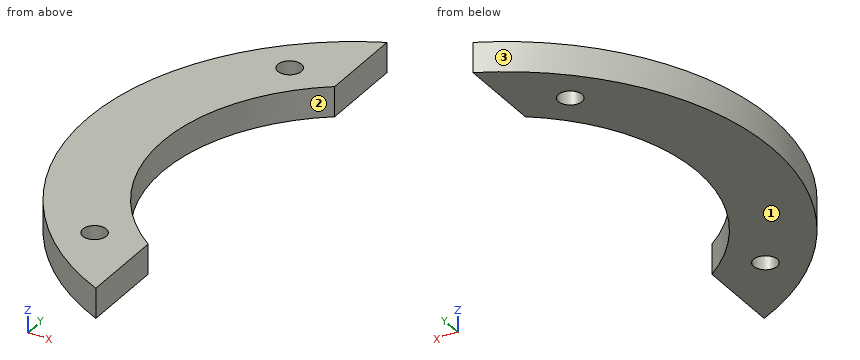
```python
from build123d import *

# Parameters (mm, degrees)
SKETCH_1_R          = 35.5
SKETCH_1_R_2        = 25.5
EXTRUDE_1_DEPTH     = 4
SKETCH_2_R          = 1.575
CUT_EXTRUDE_1_DEPTH = 51.363677388
SKETCH_3_W          = 60
SKETCH_3_H          = 80
CUT_EXTRUDE_2_DEPTH = 51.363677388


with BuildPart() as part:
    # 草图1 → 凸台-拉伸1 (new body)
    with BuildSketch(Plane.XY):
        Circle(SKETCH_1_R)
        Circle(SKETCH_1_R_2, mode=Mode.SUBTRACT)
    extrude(amount=EXTRUDE_1_DEPTH)

    # 草图2 → 切除-拉伸1 (cut, through all)
    with BuildSketch(Plane.XY.offset(4)):
        with Locations((-21.566756826, 21.566756826)):
            Circle(SKETCH_2_R)
        with Locations((21.566756826, 21.566756826)):
            Circle(SKETCH_2_R)
        with Locations((21.566756826, -21.566756826)):
            Circle(SKETCH_2_R)
        with Locations((-21.566756826, -21.566756826)):
            Circle(SKETCH_2_R)
    extrude(amount=-CUT_EXTRUDE_1_DEPTH, mode=Mode.SUBTRACT)

    # 草图3 → 切除-拉伸2 (cut, through all)
    with BuildSketch(Plane.XY.offset(4)):
        with Locations((15, 0)):
            Rectangle(SKETCH_3_W, SKETCH_3_H)
    extrude(amount=-CUT_EXTRUDE_2_DEPTH, mode=Mode.SUBTRACT)


solid = part.part
```
Source: CAD feature listing. Evaluate the final solid. Frame: model axes, mm. Face numbers are marked on the shaded views. Give positions to 0.01 mm unless a question says otherwise; leave off trailing zeros. Write each loop counter-clockwise with the first axis right and the second up, starting at its lowest first coordinate (ties: lowest second). Pieces come first, ordered by that corner, then holes. Notation, with made-up numbers: (67.25, -33) - (74.25, -33) arc R25 ccw to (74.25, 3) - close; hole circle Ø6 at (-9, -34.75). An arc over 180 degrees is marked (long way). One line per item, written item: value. Start each with the question number.
Q1. Section query D-D, the plane x = -28.25. Return the cut outline in (y, z), then the cut area to 3 significant figures.
Q2. Section query B-B, the plane y = 22.5. Return the cut outline in (x, z), then the cut area to 3 significant figures.
Q3. Section query A-A, the plane x = -17. Return the cut outline in (y, z).
Q4. Section query C-C, the plane z = 2.1. Return the cut outline in (x, y) (3 decimals).
Q5. Material intervals for probe 1 along Y at (x, z) = (-17.5, 2.45); probe 2 along X at (y, z) = (22, 2); probe 3 along Y at (x, z) = (-17.25, 3.2), sorted ascending. Write a range as from..to.
Q6. Draft query along Y for the marked faces 1, 2 and 3. Return one class per face: +Y half, -Y half, draft (parallel to the pull), parting line (faces both ways), or undercut.
Q7. First-contact query: pin 1 Ø1 at (x, z) = (-29.5, 2) entering from +Y; pin 2 Ø3 at (x, y) = (-21.57, 21.57) entering from -Z; pin 3 Ø1.5 at (y, z) = (-15.5, 1) entering from +X. Flat tips, straight axial feed; report the tip coordinate or a pass-through.
Answer:
1. outline: (-21.5, 0) - (21.5, 0) - (21.5, 4) - (-21.5, 4) - close
1. area: 172 mm2
2. outline: (-27.46, 0) - (-22.84, 0) - (-22.84, 4) - (-27.46, 4) - close; (-20.3, 0) - (-15, 0) - (-15, 4) - (-20.3, 4) - close
2. area: 39.7 mm2
3. outline: (-31.16, 0) - (-19.01, 0) - (-19.01, 4) - (-31.16, 4) - close; (19.01, 0) - (31.16, 0) - (31.16, 4) - (19.01, 4) - close
4. outline: (-15, -32.175) - (-15, -20.622) arc R25.5 cw to (-15, 20.622) - (-15, 32.175) arc R35.5 ccw to start; hole circle Ø3.15 at (-21.567, -21.567); hole circle Ø3.15 at (-21.567, 21.567)
5. probe 1: y = -30.89..-18.55, 18.55..30.89
5. probe 2: x = -27.86..-23.08, -20.05..-15
5. probe 3: y = -31.03..-18.78, 18.78..31.03
6. face 1: draft
6. face 2: undercut
6. face 3: parting line
7. pin 1: stops at y = 20.48
7. pin 2: passes through
7. pin 3: stops at x = -19.65
